from build123d import *

# Parameters (mm, degrees)
F1_DEPTH = 12.7


# Not quite as in the source:
# - a feature names something its author has since deleted; it is built from what else it names


with BuildPart() as f1:
    # F0 (on Top) → F1 (new body)
    with BuildSketch(Plane.XY):
        with BuildLine():
            Line((63.0196762211, 10.9010377465), (50.3931596336, 10.9010377465))
            Line((50.3931596336, 10.9010377465), (42.2776843256, -8.6024441122))
            Line((42.2776843256, -8.6024441122), (49.1147374354, -8.6024441122))
            Line((49.1147374354, -8.6024441122), (52.3656376201, -0.7897319333))
            Line((52.3656376201, -0.7897319333), (55.199665187, -0.7897319333))
            Line((55.199665187, -0.7897319333), (60.5922424733, -10.3281843676))
            Line((60.5922424733, -10.3281843676), (65.9258010509, -7.9737302361))
            Line((65.9258010509, -7.9737302361), (61.8239495523, -0.7183283504))
            ThreePointArc((61.8239495523, -0.7183283504), (68.5532030557, 4.4603851012), (63.0196762211, 10.9010377465))
        make_face()
        with BuildLine():
            Line((53.8841895381, 2.8597215688), (55.7706488767, 7.3933470303))
            Line((55.7706488767, 7.3933470303), (61.637538461, 7.3933470303))
            ThreePointArc((61.637538461, 7.3933470303), (63.9369023486, 5.1428976256), (61.6700313985, 2.8597215688))
            Line((61.6700313985, 2.8597215688), (53.8841895381, 2.8597215688))
        make_face(mode=Mode.SUBTRACT)
    extrude(amount=F1_DEPTH)


solid = f1.part
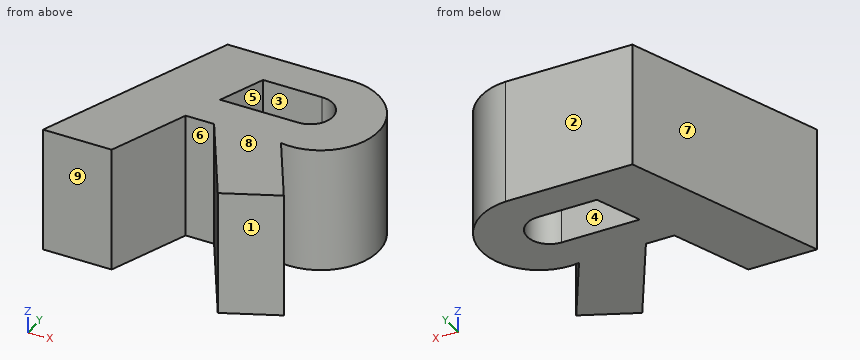
Can you work these out from the model? Positions are in its coordinate system, mm. Face numbers are marked on the shaded views. A direction names the side the tool comes from. Round coordinates to 2 decimals unless told otherwise and drop trailing zeros. Write each loop counter-clockwise with the first axis right and the second up, starting at its lowest first coordinate (ties: lowest second). Pieces come first, ordered by that corner, then holes. Notation, with made-up numbers: M 34.5,11 L 38.5,11 A21 cw 38.5,43 Z; hole C 55.5,7.25 d6. An arc over 180 degrees is marked long. Use a Markdown table: item, result.
Item 1: If I drill on line 1 along X through (y, z) = (-4.5, 2.5); line 2 along Y through (x, z) = (63.75, 5.25); line 3 along X through (y, z) = (-8.5, 12), over which ranges is the centre line in solid material (lowest first)? Write a range as [from, to].
Found:
| item | result |
|---|---|
| line 1 | x = [43.98, 50.82], [57.3, 63.96] |
| line 2 | y = [-8.93, -4.13], [-0.7, 4.23], [6.03, 10.82] |
| line 3 | x = [42.32, 49.16], [59.56, 64.73] |
Item 2: I want a section at C-C (y = 6.25). List the corners of the cut face in (x, z) for me, and give its area (3 significant figures).
Found:
| item | result |
|---|---|
| outline | M 48.46,0 L 55.29,0 L 55.29,12.7 L 48.46,12.7 Z; M 63.64,0 L 68.46,0 L 68.46,12.7 L 63.64,12.7 Z |
| area | 148 mm2 |
Item 3: We'd pull the mould along Y, two halves only. Please class the marked faces 1, 2, 3 and 4: released by +Y, released by -Y, zero draft, split by the parting line, or undercut.
Found:
| item | result |
|---|---|
| face 1 | released by -Y |
| face 2 | released by +Y |
| face 3 | undercut |
| face 4 | undercut |
Item 4: For pin 1 Ø3 at (x, z) = (65.5, 8) entering from +Y; pin 2 Ø0.9 at (x, z) = (54, 7) entering from -Y; pin 3 Ø3.5 at (x, z) = (47, 4.5) entering from -Y, each with a flat end and sliding along its axis, tell me the tip position at first contact or that it passes through.
Found:
| item | result |
|---|---|
| pin 1 | stops at y = 10.77 |
| pin 2 | stops at y = -0.79 |
| pin 3 | stops at y = -8.6 |
Item 5: I want a section at D-D (x = 66.75). List the corners of the cut face in (y, z) for me.
Found:
| item | result |
|---|---|
| outline | M 0.81,0 L 9.31,0 L 9.31,12.7 L 0.81,12.7 Z |
Item 6: I want a section at B-B (x = 56.25). List the corners of the cut face in (y, z) for me.
Found:
| item | result |
|---|---|
| outline | M -2.65,0 L 2.86,0 L 2.86,12.7 L -2.65,12.7 Z; M 7.39,0 L 10.9,0 L 10.9,12.7 L 7.39,12.7 Z |
Item 7: Which directions (+Z, -Z, +X, -X, +Y, -Y) give clear straight access to the entire face, cutting with the end or side of a thin tool? Please do the marked faces 5, 6, 7, 8 and 9.
Found:
| item | result |
|---|---|
| face 5 | +Z, -Z |
| face 6 | +Z, -Z, -Y |
| face 7 | +Z, -Z, -X, +Y |
| face 8 | +Z, +X, -X, +Y, -Y |
| face 9 | +Z, -Z, -X, -Y |
Item 8: I want a section at A-A (z = 6.5). List the corners of the cut face in (x, y) for me.
Found:
| item | result |
|---|---|
| outline | M 42.28,-8.6 L 49.11,-8.6 L 52.37,-0.79 L 55.2,-0.79 L 60.59,-10.33 L 65.93,-7.97 L 61.82,-0.72 A5.85 ccw long 63.02,10.9 L 50.39,10.9 Z; hole M 53.88,2.86 L 61.67,2.86 A2.27 ccw long 61.64,7.39 L 55.77,7.39 Z |
